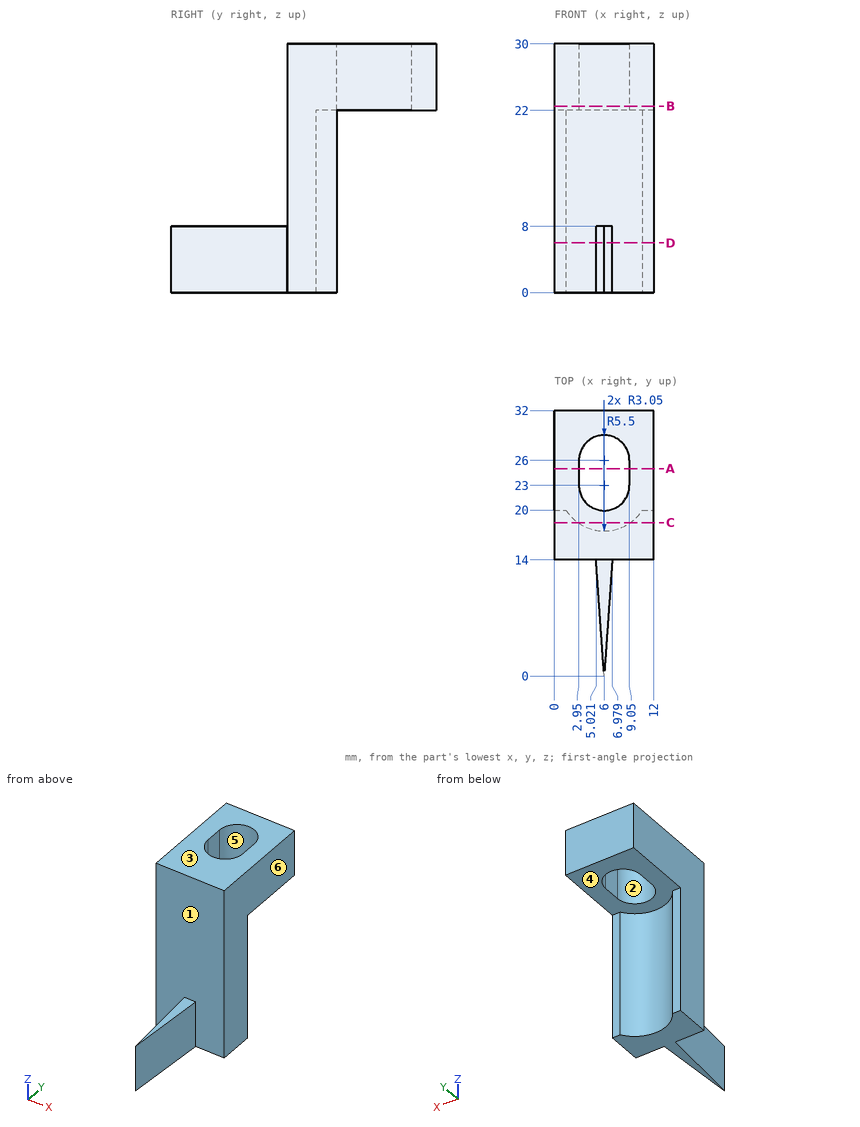
The figure shows three views and two pictorial views of one solid part (mm, origin at its lowest corner). Answer the questions. A direction names the side the tool comes from. Coordinates: 2 decimals unless noted, no trailing zeros. Order: outer loops, then holes, each group sorted by start corner. A loop starts at its lowest first (then second) coordinate and runs counter-clockwise, first axis right, second up.
Q1. A cutting plane is placed at D-D, the plane z = 6. Write down the section's boundary in (x, y), and give its area (3 significant figures).
Q2. For a pull along Y with two mould halves and no side action, classify the marked faces 1, 2 and 3 as pulls with the +Y half, pulls with the -Y half, needs draft (parallel to the pull), parting line crosses it, or undercut.
Q3. A cutting plane is placed at A-A, the plane y = 25. Write down the section's boundary in (x, z), and give its area (3 significant figures).
Q4. A cutting plane is placed at C-C, the plane y = 18.5. Write down the section's boundary in (x, z), and give its area (3 significant figures).
Q5. A cutting plane is placed at B-B, the plane z = 22.5. Write down the section's boundary in (x, y), and give its area (3 significant figures).
Q6. Consider line 1 (Y direction, x = 1, z = 5); line 2 (Z direction, x = 1.5, y = 28.5); line 3 (Z direction, x = 5.75, y = 5). Determine where each line is inside the solid, lowest interval first.
Q7. Given P1, Ø4, axis at y = 11.5, z = 7, coming from the -X side; P2, Ø2, axis at x = 10.5, y = 25, coming from the -Z side; P3, Ø1.1, axis at x = 11.5, z = 8.5, coming from the +Y side, each flat-ended and moving along its own axis, determine where each tip first touches the part or whether it passes through.
Q8. Which of the six approach directions +Z, -Z, +X, -X, +Y, -Y give full straight-line access (tool end or side, diameter ignored) to the marked faces 4, 5 and 6?
Answers follow:
1. outline: (0, 14) - (5.02, 14) - (6, 0) - (6.98, 14) - (12, 14) - (12, 20) - (10.61, 20) arc R5.5 cw to (1.39, 20) - (0, 20) - close
1. area: 69.5 mm2
2. face 1: pulls with the -Y half
2. face 2: undercut
2. face 3: needs draft
3. outline: (0, 22) - (2.95, 22) - (2.95, 30) - (0, 30) - close; (9.05, 22) - (12, 22) - (12, 30) - (9.05, 30) - close
3. area: 47.2 mm2
4. outline: (0, 0) - (2.84, 0) - (2.84, 22) - (9.16, 22) - (9.16, 0) - (12, 0) - (12, 30) - (0, 30) - close
4. area: 221 mm2
5. outline: (0, 14) - (12, 14) - (12, 32) - (0, 32) - close; hole (2.95, 23) arc R3.05 ccw to (9.05, 23) - (9.05, 26) arc R3.05 ccw to (2.95, 26) - close
5. area: 168 mm2
6. line 1: y = 14 to 20
6. line 2: z = 22 to 30
6. line 3: z = 0 to 8
7. P1: stops at x = 5.06
7. P2: stops at z = 22
7. P3: stops at y = 20
8. face 4: -Z, +Y
8. face 5: +Z, -Z
8. face 6: +Z, -Z, +X, +Y, -Y
